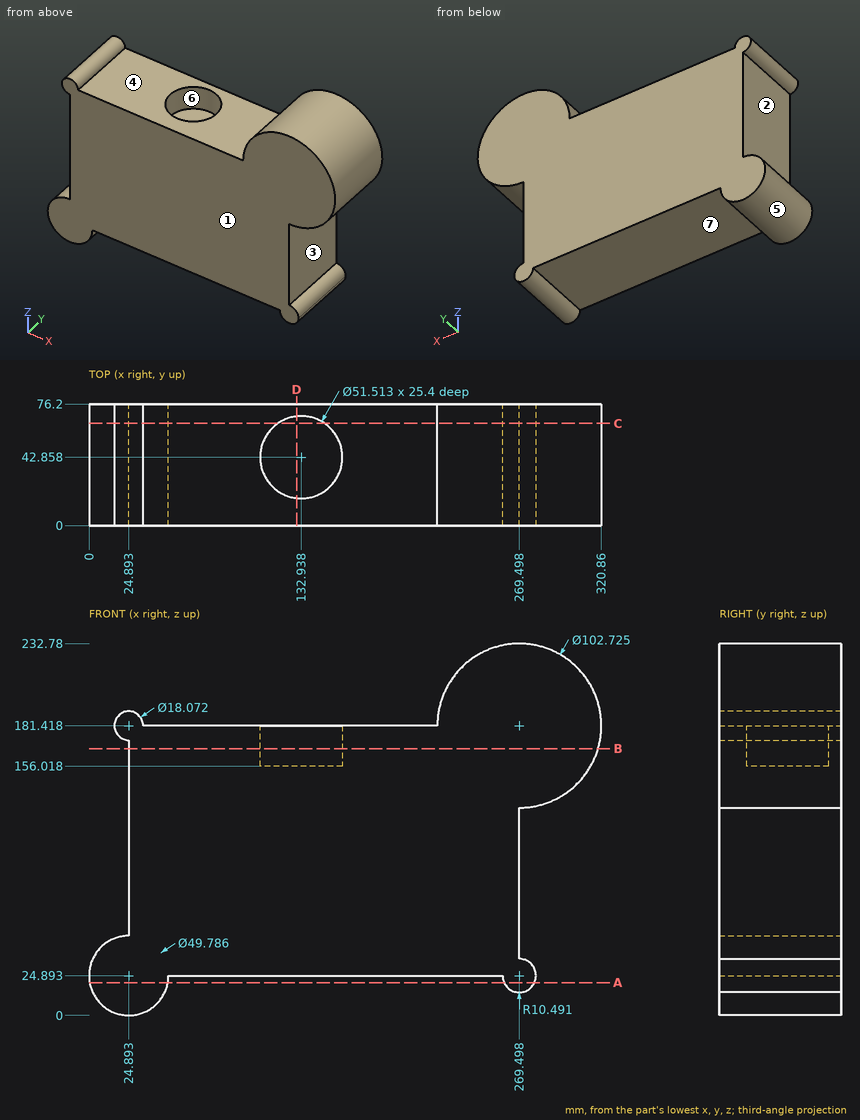
Geometry: see drawing. Coordinates: mm, zero at the bounding-box minimum. A direction names the side the tool comes from. Give positions to 0.01 mm unless a question says otherwise; leave off trailing zeros. Loops run counter-clockwise (first coordinate to the right, second up) from the corner with the lowest first, then second, coordinate; pieces in that order, holes last. Notation, with made-up numbers: (20, 41) - (32, 41) arc R15 cw to (32, 50) - close; hole circle Ø1 at (82, -19). An arc over 180 degrees is marked (long way). Use CSV: the item, a comma, the result in double quotes. Start each with the question number.
Item 1: Section A-A on z = 20.5. Return loops of the section in (x, y) (1 decimal).
Item 2: Section D-D on x = 130. Return loops of the section in (y, z), then the cut area to 3 significant figures.
Item 3: Section C-C on y = 64. Return loops of the section in (x, z) (1 decimal), then the cut area to 3 significant figures.
Item 4: Mould query, pull axis Z, two halves, no side actions, for the marked faces 1, 2, 3 and 4. Classes: pulls with the +Z half, pulls with the -Z half, needs draft (parallel to the pull), parting line crosses it, or undercut.
Item 5: Line query: line 1 (X direction, y = 16, z = 66.5); line 2 (Z direction, x = 99, y = 30.5); line 3 (Z direction, x = 130, y = 65). Output: solid intervals per line, ascending.
Item 6: Reachability of the marked faces 5, 6 and 7 from +Z, -Z, +X, -X, +Y, -Y: full face, straight path, thin tool, end or side. Return the list, or none.
Item 7: Contact query for flat-ended pins moving along their axis: P1, Ø8, axis at x = 111.5, z = 126.5, coming from the -Y side; P2, Ø23, axis at y = 40, z = 116, coming from the -X side; P3, Ø1, axis at x = 132, y = 47.5, coming from the +Z side; P4, Ø10, axis at y = 54, z = 195, coming from the +X side. Output: stop coordinate, or through.
Item 8: Section B-B on z = 167. Return loops of the section in (x, y) (1 decimal).
Ans:
1,outline,"(0.4, 0) - (49.4, 0) - (49.4, 76.2) - (0.4, 76.2) - close; (260, 0) - (279, 0) - (279, 76.2) - (260, 76.2) - close"
2,outline,"(0, 24.89) - (76.2, 24.89) - (76.2, 181.42) - (68.45, 181.42) - (68.45, 156.02) - (17.27, 156.02) - (17.27, 181.42) - (0, 181.42) - close"
2,area,"10,600 mm2"
3,outline,"(24.9, 49.8) arc R24.9 ccw (long way) to (49.8, 24.9) - (259, 24.9) arc R10.5 ccw (long way) to (269.5, 35.4) - (269.5, 130.1) arc R51.4 ccw (long way) to (218.1, 181.4) - (147.6, 181.4) - (147.6, 156) - (118.2, 156) - (118.2, 181.4) - (33.9, 181.4) arc R9 ccw (long way) to (24.9, 172.4) - close"
3,area,"45,700 mm2"
4,face 1,"needs draft"
4,face 2,"undercut"
4,face 3,"undercut"
4,face 4,"pulls with the +Z half"
5,line 1,"x = 24.89 to 269.5"
5,line 2,"z = 24.89 to 181.42"
5,line 3,"z = 24.89 to 156.02"
6,face 5,"+Y, -Y"
6,face 6,"+Z"
6,face 7,"-Z, +Y, -Y"
7,P1,"stops at y = 0"
7,P2,"stops at x = 24.89"
7,P3,"stops at z = 156.02"
7,P4,"stops at x = 320.14"
8,outline,"(24.9, 0) - (318.8, 0) - (318.8, 76.2) - (24.9, 76.2) - close; hole circle Ø51.5 at (132.9, 42.9)"
